Study the drawing (mm; zero at the part's minimum x, y, z) and answer. Round coordinates to 2 decimals unless told otherwise and drop trailing zeros. Order: outer loops, then holes, each group sorted by start corner. A loop starts at its lowest first (then second) coordinate and runs counter-clockwise, first axis right, second up. Notation, with made-up numbers: (74, 35.5) -> (133, 35.5) arc R28 cw to (133, 59.5) -> close; hole circle Ø2 at (86.5, 4.25). An arc over 180 degrees is marked (long way). Use one line per item in the form item = value.
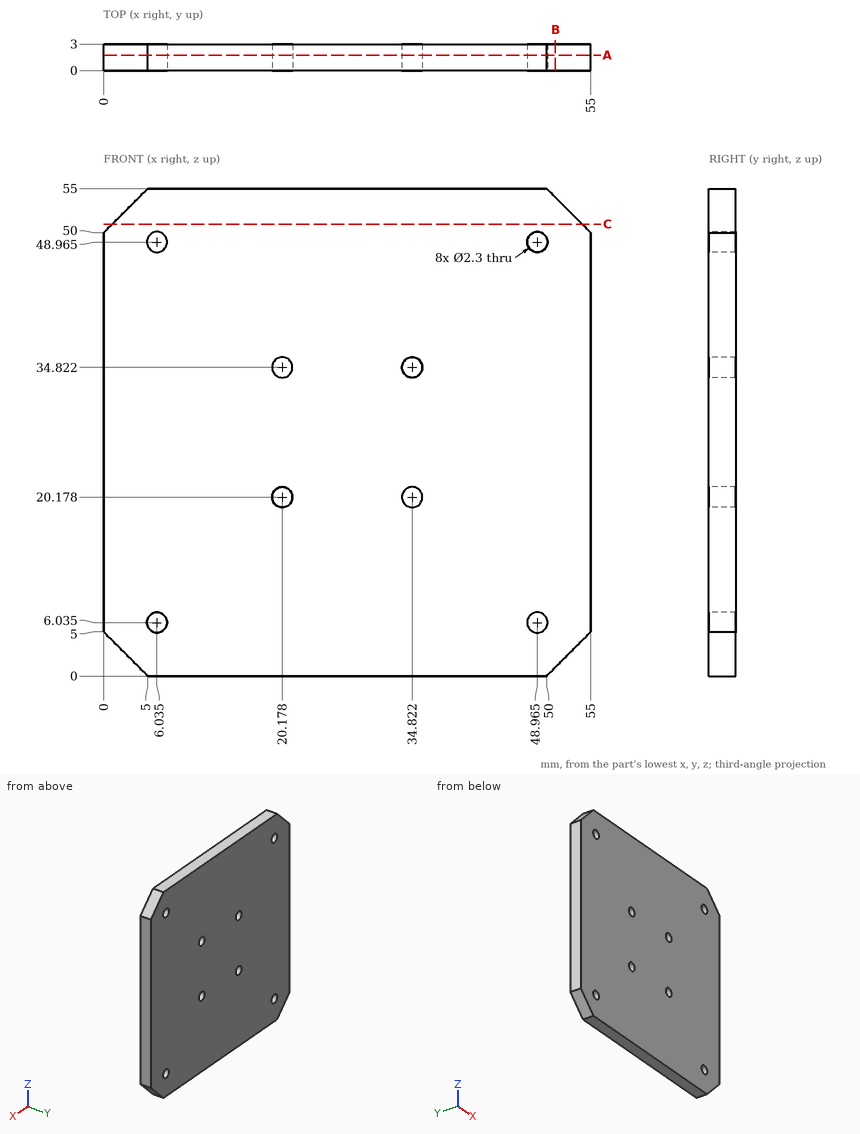
Item 1: Consider line 1 along Z through (x, y) = (34.5, 1.8) (1 decimal); line 2 along X through (y, z) = (1.4, 5.5) (1 decimal); line 3 along X through (y, z) = (2.8, 5) (1 decimal). Determine where each line is inside the solid, lowest interval first.
Findings:
line_1 = 0 to 19.1, 21.3 to 33.7, 35.9 to 55
line_2 = 0 to 5, 7.1 to 47.9, 50 to 55
line_3 = 0 to 5.5, 6.5 to 48.5, 49.5 to 55
Item 2: The part is cut by section A-A, the plane y = 1.75. Give the number of separate pieces and of enclosed holes in the cut face, and give its area (3 significant figures).
Findings:
separate_pieces = 1
enclosed_holes = 8
area = 2,940 mm^2
Item 3: The part is cut by section B-B, the plane x = 51. Give the vertices of the cut face in (y, z).
Findings:
outline = (0, 1) -> (3, 1) -> (3, 54) -> (0, 54) -> close
Item 4: The part is cut by section C-C, the plane z = 51. Give the vertices of the cut face in (x, y), and give its area (3 significant figures).
Findings:
outline = (1, 0) -> (54, 0) -> (54, 3) -> (1, 3) -> close
area = 159 mm^2
Item 5: A flat-ended cylindrical pin translates along its axis: P1, Ø3.5, axis at x = 6.04, z = 6.04, coming from the +Y side. Find the tip coordinate at first contact, or state that the pin passes through.
Findings:
P1 = 3
